Geometry check sheet. Reference: the model listing, model coordinates, mm. Face numbers are marked on the shaded views. Round coordinates to 2 decimals unless told otherwise and drop trailing zeros. Loops run counter-clockwise (first coordinate to the right, second up) from the corner with the lowest first, then second, coordinate; pieces in that order, holes last.
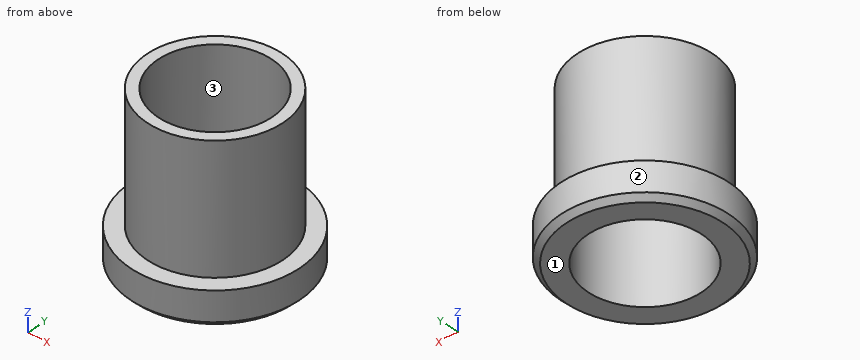
```python
from build123d import *

# Parameters (mm, degrees)
F0_R     = 11.684
F0_R_2   = 7.8867
F1_DEPTH = 4.826
F2_R     = 9.40435
F2_R_2   = 7.8867
F3_DEPTH = 17.526
F4_SIZE2 = 0.762
F4_SIZE  = 0.762


with BuildPart() as f1:
    # F0 (on Top) → F1 (new body)
    with BuildSketch(Plane.XY):
        Circle(F0_R)
        Circle(F0_R_2, mode=Mode.SUBTRACT)
    extrude(amount=F1_DEPTH)

    # F2 (on face) → F3 (join)
    with BuildSketch(Plane.XY.offset(4.826)):
        Circle(F2_R)
        Circle(F2_R_2, mode=Mode.SUBTRACT)
    extrude(amount=F3_DEPTH)

    # F4
    f4_edges = [f1.edges().sort_by_distance(p)[0] for p in [
        (-11.684, 0, 0),
    ]]
    chamfer(f4_edges, length=F4_SIZE, length2=F4_SIZE2)


solid = f1.part
```
1) Mould release check, pull along Y, two halves, no side actions. Record for the marked faces 1, 2 and 3: +Y half, -Y half, draft (parallel to the pull), parting line (faces both ways), or undercut.
Report:
face 1: draft
face 2: parting line
face 3: undercut
2) Sectioned sample at C-C, the plane z = 14.75. Record the cut outline in (x, y), then the cut area to 3 significant figures.
Report:
outline: circle Ø18.81 at (0, 0); hole circle Ø15.77 at (0, 0)
area: 82.4 mm2
3) Scan lines: line 1 along Y through (x, z) = (0, 15.5); line 2 along X through (y, z) = (-2.75, 14); line 3 along Y through (x, z) = (1.25, 21.75). Record each from-to range of solid material in increasing order.
Report:
line 1: y = -9.4 to -7.89, 7.89 to 9.4
line 2: x = -8.99 to -7.39, 7.39 to 8.99
line 3: y = -9.32 to -7.79, 7.79 to 9.32
4) Gauge pin test, flat ends, axial feed: pin 1 (1.5 mm diameter, centred on y = 5, z = 13.5, fed in from -X); pin 2 (4 mm diameter, centred on y = 4.5, z = 9, fed in from +X); pin 3 (12.5 mm diameter, centred on x = 0, y = 0, fed in from -Z); pin 4 (3 mm diameter, centred on x = -3, z = 4.5, fed in from -Y). Record the tip position at first contact, or that the pin passes through.
Report:
pin 1: stops at x = -8.39
pin 2: stops at x = 9.07
pin 3: passes through
pin 4: stops at y = -11.59
5) Sectioned sample at A-A, the plane x = 0. Record the cut outline in (y, z), then the cut area to 3 significant figures.
Report:
outline: (-11.68, 0.76) - (-10.92, 0) - (-7.89, 0) - (-7.89, 22.35) - (-9.4, 22.35) - (-9.4, 4.83) - (-11.68, 4.83) - close; (7.89, 0) - (10.92, 0) - (11.68, 0.76) - (11.68, 4.83) - (9.4, 4.83) - (9.4, 22.35) - (7.89, 22.35) - close
area: 89.3 mm2
